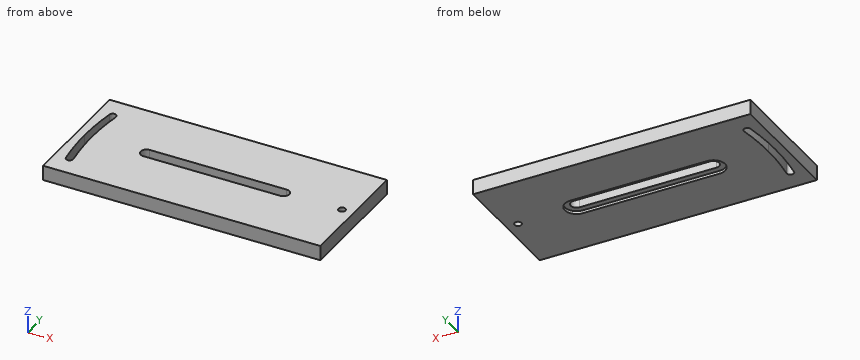
```python
from build123d import *

# Parameters (mm, degrees)
F0_W     = 236.99978
F0_H     = 105.4
F1_DEPTH = 12.7
F2_R     = 3
F3_DEPTH = 12.701
F4_DEPTH = 2.54


with BuildPart() as f1:
    # F0 (on Top) → F1 (new body)
    with BuildSketch(Plane.XY):
        with Locations((0.00011, 0)):
            Rectangle(F0_W, F0_H)
    extrude(amount=F1_DEPTH)

    # F2 (on Top) → F3 (cut, through all)
    with BuildSketch(Plane.XY):
        with BuildLine():
            Line((0, 5), (-58.49989, 5))
            ThreePointArc((-58.49989, 5), (-63.49989, 0), (-58.49989, -5))
            Line((-58.49989, -5), (0, -5))
            Line((0, -5), (58.50011, -5))
            ThreePointArc((58.50011, -5), (63.50011, 0), (58.50011, 5))
            Line((58.50011, 5), (0, 5))
        make_face()
        with BuildLine():
            ThreePointArc((-108.791217, 34.415555), (-106.297456, 30.983186), (-102.865087, 33.476947))
            ThreePointArc((-102.865087, 33.476947), (-102.8374, 33.710873), (-102.828152, 33.946251))
            ThreePointArc((-102.828152, 33.946251), (-105.592775, 36.937003), (-108.791217, 34.415555))
        make_face()
        with BuildLine():
            ThreePointArc((-102.865087, -33.476947), (-104.84009, -16.790232), (-105.49978, 0))
            ThreePointArc((-105.49978, 0), (-104.84009, 16.790232), (-102.865087, 33.476947))
            ThreePointArc((-102.865087, 33.476947), (-106.297456, 30.983186), (-108.791217, 34.415555))
            ThreePointArc((-108.791217, 34.415555), (-110.821594, 17.260987), (-111.49978, 0))
            ThreePointArc((-111.49978, 0), (-110.821594, -17.260987), (-108.791217, -34.415554))
            ThreePointArc((-108.791217, -34.415554), (-106.297456, -30.983186), (-102.865087, -33.476947))
        make_face()
        with BuildLine():
            ThreePointArc((-102.828152, -33.946251), (-102.8374, -33.710873), (-102.865087, -33.476947))
            ThreePointArc((-102.865087, -33.476947), (-106.297456, -30.983186), (-108.791217, -34.415554))
            ThreePointArc((-108.791217, -34.415554), (-105.592775, -36.937003), (-102.828152, -33.946251))
        make_face()
        with Locations((108.50004, 0)):
            Circle(F2_R)
    extrude(amount=F3_DEPTH, mode=Mode.SUBTRACT)

    # F2 (on Top) → F4 (cut)
    with BuildSketch(Plane.XY):
        with BuildLine():
            Line((0, 10), (-58.49989, 10))
            ThreePointArc((-58.49989, 10), (-68.49989, 0), (-58.49989, -10))
            Line((-58.49989, -10), (0, -10))
            Line((0, -10), (58.50011, -10))
            ThreePointArc((58.50011, -10), (68.50011, 0), (58.50011, 10))
            Line((58.50011, 10), (0, 10))
        make_face()
        with BuildLine():
            ThreePointArc((-58.49989, -5), (-63.49989, 0), (-58.49989, 5))
            Line((-58.49989, 5), (0, 5))
            Line((0, 5), (58.50011, 5))
            ThreePointArc((58.50011, 5), (63.50011, 0), (58.50011, -5))
            Line((58.50011, -5), (0, -5))
            Line((0, -5), (-58.49989, -5))
        make_face(mode=Mode.SUBTRACT)
    extrude(amount=F4_DEPTH, mode=Mode.SUBTRACT)


solid = f1.part
```
Input: part model. Units: mm. Frame: model coordinates. Round coordinates to 2 decimals unless told otherwise and drop trailing zeros. Order: outer loops, then holes, each group sorted by start corner. A loop starts at its lowest first (then second) coordinate and runs counter-clockwise, first axis right, second up. Notation, with made-up numbers: (89.5, 9.25) - (138.5, 9.25) arc R23 cw to (138.5, 41.25) - close; hole circle Ø9 at (41, 23.5). An arc over 180 degrees is marked (long way). Answer in a Markdown table with one row per item.
Item 1: Section query D-D (y = -20.5). Return the cut outline in (x, z).
Model answer:
| item | result |
|---|---|
| outline | (-118.5, 0) - (-110.54, 0) - (-110.54, 12.7) - (-118.5, 12.7) - close; (-104.52, 0) - (118.5, 0) - (118.5, 12.7) - (-104.52, 12.7) - close |
Item 2: Section query B-B (z = 4.5). Return the cut outline in (x, y), then the cut area to 3 significant figures.
Model answer:
| item | result |
|---|---|
| outline | (-118.5, -52.7) - (118.5, -52.7) - (118.5, 52.7) - (-118.5, 52.7) - close; hole (-111.5, 0) arc R220 ccw to (-108.79, -34.42) arc R3 ccw to (-102.83, -33.95) arc R3 ccw to (-102.87, -33.48) arc R214 cw to (-105.5, 0) arc R214 cw to (-102.87, 33.48) arc R3 ccw to (-102.83, 33.95) arc R3 ccw to (-108.79, 34.42) arc R220 ccw to start; hole (-58.5, -5) - (58.5, -5) arc R5 ccw to (58.5, 5) - (-58.5, 5) arc R5 ccw to start; hole circle Ø6 at (108.5, 0) |
| area | 23,300 mm² |
Item 3: Section query C-C (y = 28.5). Return the cut outline in (x, z).
Model answer:
| item | result |
|---|---|
| outline | (-118.5, 0) - (-109.65, 0) - (-109.65, 12.7) - (-118.5, 12.7) - close; (-103.59, 0) - (118.5, 0) - (118.5, 12.7) - (-103.59, 12.7) - close |
Item 4: Pin query (flat end, axial travel): pin 1 (10 mm diameter, centred on x = -2, y = -1, fed in from -Z); pin 2 (3.5 mm diameter, centred on x = 108.5, y = 0, fed in from +Z). Return the tip coordinate at first contact, or that it passes through.
Model answer:
| item | result |
|---|---|
| pin 1 | stops at z = 2.54 |
| pin 2 | passes through |
Item 5: Section query A-A (x = 45). Return the cut outline in (y, z), then the cut area to 3 significant figures.
Model answer:
| item | result |
|---|---|
| outline | (-52.7, 0) - (-10, 0) - (-10, 2.54) - (-5, 2.54) - (-5, 12.7) - (-52.7, 12.7) - close; (5, 2.54) - (10, 2.54) - (10, 0) - (52.7, 0) - (52.7, 12.7) - (5, 12.7) - close |
| area | 1,190 mm² |
Item 6: Line query: line 1 (X direction, y = 0, z = 8.75); line 2 (Y direction, x = 26.5, z = 2.75); line 3 (X direction, y = 19.5, z = 3.5). Output: solid intervals per line, ascending.
Model answer:
| item | result |
|---|---|
| line 1 | x = -118.5 to -111.5, -105.5 to -63.5, 63.5 to 105.5, 111.5 to 118.5 |
| line 2 | y = -52.7 to -5, 5 to 52.7 |
| line 3 | x = -118.5 to -110.63, -104.61 to 118.5 |
